Can you work these out from the model? Positions are in its coordinate system, mm. Face numbers are marked on the shaded views. A direction names the side the tool comes from. Give positions to 0.01 mm unless a question says otherwise; leave off trailing zeros. Order: outer loops, then holes, each group sorted by start corner. A loop starts at its lowest first (then second) coordinate and runs counter-clockwise, first axis right, second up.
Item 1: I want a section at B-B, the plane z = -23. Write out the boundary of the cut face in (x, y).
Item 2: I'm going to push flat-ended pins straight in: pin 1 Ø3 at (x, y) = (2.5, 45.5) entering from +Z; pin 2 Ø12 at (x, y) = (13, -17.5) entering from -Z; pin 3 Ø8 at (y, z) = (8.5, -8.5) entering from +X; pin 4 Ø15 at (y, z) = (31, -31.5) entering from +X (3 decimals). Where does each tip first touch, or does it pass through?
Item 3: I want a section at D-D, the plane z = -7.5. Write out the boundary of the cut face in (x, y), then the cut area to 3 significant figures.
Item 4: If I drill on line 1 along Y through (x, z) = (-7.5, -47); line 2 along Z through (x, y) = (-13.5, 40); line 3 along X through (y, z) = (4.5, -21), over which ranges is the centre line in solid material (lowest first)?
Item 5: Which directions (+Z, -Z, +X, -X, +Y, -Y) give clear straight access to the entire face, cutting with the end or side of a thin tool? Please do the marked faces 1, 2 and 3.
Item 6: If we mould it in two halves opening along X, with no side actions, what happens to the marked faces 4, 5, 6 and 7? For each: +X half, -X half, draft (parallel to the pull), parting line (faces both ways), or undercut.
Item 7: I want a section at A-A, the plane x = 22. Write out the boundary of the cut face in (y, z).
Item 8: I want a section at C-C, the plane y = 44.5. Write out the boundary of the cut face in (x, z), then the cut area to 3 significant figures.
```python
from build123d import *

# Parameters (mm, degrees)
F1_W          = 80
F1_H          = 60
F2_DEPTH      = 50
F0_W          = 80
F0_H          = 40
F3_DEPTH      = 10
F4_W          = 30.096792616
F4_H          = 78.1024228781
F5_DEPTH      = 50
F5_DEPTH_BACK = 50
F7_W          = 62.432192266
F7_H          = 30.8429924771
F7_W_2        = 62.183458358
F7_H_2        = 28.1069204211
F8_DEPTH      = 25


with BuildPart() as f2:
    # F1 (on Front) → F2 (new body)
    with BuildSketch(Plane.XZ):
        with Locations((-0.1705093682, -30)):
            Rectangle(F1_W, F1_H)
    extrude(amount=-F2_DEPTH)

    # F0 (on Top) → F3 (join)
    with BuildSketch(Plane.XY):
        with Locations((0.3269584477, -20)):
            Rectangle(F0_W, F0_H)
    extrude(amount=-F3_DEPTH)

    # F4 (on Right) → F5 (cut, two sides)
    with BuildSketch(Plane.YZ) as f5_sk:
        with Locations((24.8733828776, -9.576250799)):
            Rectangle(F4_W, F4_H)
    extrude(amount=-F5_DEPTH, mode=Mode.SUBTRACT)
    extrude(f5_sk.sketch, amount=F5_DEPTH_BACK, mode=Mode.SUBTRACT)

    # F7 (on offset) → F8 (cut)
    with BuildSketch(Plane.XZ.offset(-50)):
        with Locations((-0.7462017238, 2.8604404069)):
            Rectangle(F7_W, F7_H)
        with Locations((-0.8705686778, -32.300055027)):
            Rectangle(F7_W_2, F7_H_2)
    extrude(amount=F8_DEPTH, mode=Mode.SUBTRACT)


solid = f2.part
```
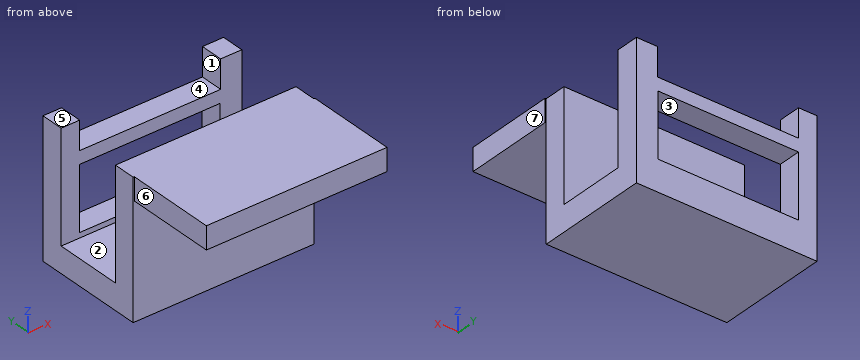
Results list:
1. outline: (-40.17, 0) - (39.83, 0) - (39.83, 9.82) - (-40.17, 9.82) - close; (-40.17, 39.92) - (-31.96, 39.92) - (-31.96, 50) - (-40.17, 50) - close; (30.22, 39.92) - (39.83, 39.92) - (39.83, 50) - (30.22, 50) - close
2. pin 1: stops at z = -12.56
2. pin 2: stops at z = -10
2. pin 3: stops at x = 39.83
2. pin 4: passes through
3. outline: (-40.17, 0) - (-39.67, 0) - (-39.67, -40) - (40.33, -40) - (40.33, 0) - (39.83, 0) - (39.83, 9.82) - (-40.17, 9.82) - close; (-40.17, 39.92) - (-31.96, 39.92) - (-31.96, 50) - (-40.17, 50) - close; (30.47, 39.92) - (39.83, 39.92) - (39.83, 50) - (30.47, 50) - close
3. area: 4,160 mm2
4. line 1: y = 0 to 9.82, 39.92 to 50
4. line 2: z = -60 to -46.35, -18.25 to -12.56
4. line 3: x = -40.17 to 39.83
5. face 1: +Z, +Y
5. face 2: +Z, +X, -X
5. face 3: +Y
6. face 4: undercut
6. face 5: draft
6. face 6: -X half
6. face 7: +X half
7. outline: (-40, -10) - (0, -10) - (0, -60) - (50, -60) - (50, -46.35) - (39.92, -46.35) - (39.92, -48.63) - (9.82, -48.63) - (9.82, 0) - (-40, 0) - close; (39.92, -18.25) - (50, -18.25) - (50, -12.56) - (39.92, -12.56) - close
8. outline: (-40.17, -60) - (39.83, -60) - (39.83, 0) - (30.47, 0) - (30.47, -12.56) - (-31.96, -12.56) - (-31.96, 0) - (-40.17, 0) - close; hole (-31.96, -46.35) - (30.22, -46.35) - (30.22, -18.25) - (-31.96, -18.25) - close
8. area: 2,270 mm2
